Autodesk Inventor part; units mm, degrees
ref_plane "YZ Plane" through (0, 0, 0) normal (1, 0, 0) x (0, 1, 0)
ref_plane "XZ Plane" through (0, 0, 0) normal (0, 1, 0) x (-1, 0, 0)
ref_plane "XY Plane" through (0, 0, 0) normal (0, 0, 1) x (1, 0, 0)
sketch "Sketch1" plane through (0, 0, 0) normal (0, 1, 0) x (-1, 0, 0)
  line L0 (2.54, 0) -> (19.05, 0)
  line L1 (21.59, -2.54) -> (21.59, -25.4)
  line L2 (19.05, -27.94) -> (2.54, -27.94)
  line L3 (0, -25.4) -> (0, -2.54)
  arc A0 (21.59, -2.54) -> (19.05, 0) centre (19.05, -2.54) ccw
  arc A1 (2.54, 0) -> (0, -2.54) centre (2.54, -2.54) ccw
  arc A2 (0, -25.4) -> (2.54, -27.94) centre (2.54, -25.4) ccw
  arc A3 (19.05, -27.94) -> (21.59, -25.4) centre (19.05, -25.4) ccw
  circle A4 centre (19.05, -2.54) radius 0.635
  circle A5 centre (2.54, -2.54) radius 0.635
  circle A6 centre (2.54, -25.4) radius 0.635
  circle A7 centre (19.05, -25.4) radius 0.635
  point P0 (0, 0)
  point P1 (21.59, -27.94)
  point P2 (21.59, 0)
  point P3 (0, -27.94)
  dimension "d0" = 21.59
  dimension "d1" = 27.94
  dimension "d2" = 2.54
  dimension "d3" = 1.27
  dimension "d4" = 1.27
  dimension "d5" = 1.27
  dimension "d6" = 1.27
extrude "Extrusion1" add sketch "Sketch1" along normal blind 1.27
sketch "Sketch2" plane through (0, 1.27, 0) normal (0, 1, 0) x (1, 0, 0)
  line L0 (-19.05, 0) -> (-2.54, 0) construction
  line L1 (-10.795, 0) -> (-10.795, 27.94) construction
  line L2 (-2.54, 27.94) -> (-19.05, 27.94) construction
  line L3 (-13.97, 27.94) -> (-7.62, 27.94) construction
  line L4 (-7.62, 27.94) -> (-7.62, 21.59) construction
  line L5 (-7.62, 21.59) -> (-13.97, 21.59) construction
  line L6 (-13.97, 21.59) -> (-13.97, 27.94) construction
  line L7 (-13.97, 21.59) -> (-7.62, 21.59) construction
  line L8 (-7.62, 21.59) -> (-7.62, 27.94) construction
  line L9 (-7.62, 27.94) -> (-13.97, 27.94) construction
  line L10 (-13.97, 27.94) -> (-13.97, 21.59) construction
  line L11 (-13.97, 21.59) -> (-7.62, 21.59)
  line L12 (-7.62, 21.59) -> (-7.62, 27.94)
  line L13 (-7.62, 27.94) -> (-13.97, 27.94)
  line L14 (-13.97, 27.94) -> (-13.97, 21.59)
  point P0 (0, 0)
  dimension "d9" = 6.35
  dimension "d10" = 6.35
  dimension "d11" = 3.175
extrude "Extrusion2" add sketch "Sketch2" along normal blind 6.35
sketch "Sketch3" plane through (0, 1.27, 0) normal (0, 1, 0) x (1, 0, 0)
  line L0 (-18.295, 10) -> (-3.295, 10)
  line L1 (-3.295, 10) -> (-3.295, 0)
  line L2 (-3.295, 0) -> (-18.295, 0)
  line L3 (-18.295, 0) -> (-18.295, 10)
  line L4 (-7.62, 27.94) -> (-13.97, 27.94) construction
  line L5 (-10.795, 27.94) -> (-10.795, 0) construction
  line L6 (-2.54, 0) -> (-19.05, 0) construction
  line L7 (-10.795, 10) -> (-10.795, 0) construction
  line L8 (-19.05, 0) -> (-2.54, 0) construction
  point P0 (0, 0)
  dimension "d14" = 15
  dimension "d15" = 10
extrude "Extrusion3" add sketch "Sketch3" along normal blind 8
equation "\"d4\" = d3"
equation "\"d5\" = d3"
equation "\"d6\" = d3"
equation "\"d11\" = 0.5 * d10"
properties part number "Adafruit-PowerBoost500"
Design review of the part built by this model. Coordinates are the model's own, in mm. A direction names the side the tool comes from. Round coordinates to 2 decimals unless told otherwise and drop trailing zeros. Write each loop counter-clockwise with the first axis right and the second up, starting at its lowest first coordinate (ties: lowest second). Pieces come first, ordered by that corner, then holes. Notation, with made-up numbers: (-17.75, 33.5) -> (-4.75, 33.5) arc R34 cw to (-4.75, 63.5) -> close; hole circle Ø6 at (-29.5, -20.75). An arc over 180 degrees is marked (long way). Write item = value, one per line. Start each with the question number.
1) Tool access review of faces 1 (the face through (-13.97, 4, -25)), 2 (the face through (-3.295, 5, -5)), 3 (the face through (-11, 5, -10)): name each direction out of +Z, -Z, +X, -X, +Y, -Y from which nothing blocks a thin tool from reaching the whole face with its end or side.
2) Take a section at B-B, the plane x = -9. State the section outline as (y, z) points.
3) Wall thickness on probe 1 along Z at (x, y) = (-2.54, 0.9) (3 decimals); probe 2 along Z at (x, y) = (-8.75, 4.75); probe 3 along X at (y, z) = (7.5, -8.75) (3 decimals): over which ranges is each line inside the solid? List them lowest first. Write a range as from..to.
4) Take a section at C-C, the plane z = -5. State the section outline as (x, y) points (3 decimals).
5) Clearance check with flat-ended pins moving along their axes: pin 1 (2 mm diameter, centred on x = -14.5, y = 3.5, fed in from +Z); pin 2 (3 mm diameter, centred on y = 3.5, z = -26.5, fed in from -X); pin 3 (4 mm diameter, centred on y = 6.5, z = -6, fed in from -X) (3 decimals); pin 4 (3 mm diameter, centred on x = -9.5, z = -25.5, fed in from +Y). State where each tip first meets the part, or that it passes through.
6) Take a section at D-D, the plane x = -16.5. State the section outline as (y, z) points, plus the area to 3 significant figures.
7) Mouldability with a two-part tool opening along Z and no side actions: class faces 4 (the face through (-21.59, 1, -14)), 5 (the face through (-2.04, 0.63, -2.15)), 6 (the face through (-11, 5, 0)), 7 (the face through (-11, 3, -27.94)) as +Z half, -Z half, draft (parallel to the pull), parting line (faces both ways), or undercut.
8) Take a section at A-A, the plane y = 4. State the section outline as (x, z) points (3 decimals).
Results list:
q1.face_1 = -Z, -X, +Y
q1.face_2 = +Z, -Z, +X, +Y
q1.face_3 = +X, -X, +Y
q2.outline = (0, -27.94) -> (7.62, -27.94) -> (7.62, -21.59) -> (1.27, -21.59) -> (1.27, -10) -> (9.27, -10) -> (9.27, 0) -> (0, 0) -> close
q3.probe_1 = -27.94..-26.035, -24.765..-3.175, -1.905..0
q3.probe_2 = -27.94..-21.59, -10..0
q3.probe_3 = -18.295..-3.295
q4.outline = (-21.59, 0) -> (0, 0) -> (0, 1.27) -> (-3.295, 1.27) -> (-3.295, 9.27) -> (-18.295, 9.27) -> (-18.295, 1.27) -> (-21.59, 1.27) -> close
q5.pin_1 = 0
q5.pin_2 = -13.97
q5.pin_3 = -18.295
q5.pin_4 = 7.62
q6.outline = (0, -27.94) -> (1.27, -27.94) -> (1.27, -10) -> (9.27, -10) -> (9.27, 0) -> (0, 0) -> close
q6.area = 115 mm²
q7.face_4 = draft
q7.face_5 = undercut
q7.face_6 = +Z half
q7.face_7 = -Z half
q8.outline = (-18.295, -10) -> (-3.295, -10) -> (-3.295, 0) -> (-18.295, 0) -> close; (-13.97, -27.94) -> (-7.62, -27.94) -> (-7.62, -21.59) -> (-13.97, -21.59) -> close
